The figure shows three views and two pictorial views of one solid part (mm, origin at its lowest corner). Answer the questions. Coordinates: 2 decimals unless noted, no trailing zeros. Write each loop counter-clockwise with the first axis right and the second up, starting at its lowest first coordinate (ties: lowest second). Pieces come first, ordered by that corner, then holes. Notation, with made-up numbers: (4, 7.25) - (33, 7.25) arc R29 cw to (33, 33.25) - close; hole circle Ø3 at (12, 72.25). An arc over 180 degrees is marked (long way). Use a Markdown table: item, result. Add a question column.
(1) Find the intervals of material crossed by line 1 (X direction, y = 6.25, z = 23) (1 decimal); line 2 (X direction, y = 1.5, z = 34.5); line 3 (Y direction, x = 40.5, z = 35.5), in increasing order. Write a range as from..to.
(2) For a pull along Z with two mould halves and no side action, classify the marked faces 1, 2, 3 and 4 as released by +Z, released by -Z, zero draft, split by the parting line, or undercut.
(3) The part is cut by section D-D, the plane z = 15. Give the vertices of the cut face in (x, y), then the cut area to 3 significant figures.
(4) Given pin 1 Ø3.5 at (x, z) = (17.02, 15.4) entering from -Y; pin 2 Ø1 at (x, z) = (36, 26) entering from +Y (3 decimals); pin 3 Ø3.5 at (x, z) = (29.15, 36.4) entering from +Y, each flat-ended and moving along its own axis, determine where each tip first touches the part or whether it passes through.
(5) The part is cut by section C-C, the plane x = 29.15. Give the vertices of the cut face in (y, z) (1 decimal), then the cut area to 3 significant figures.
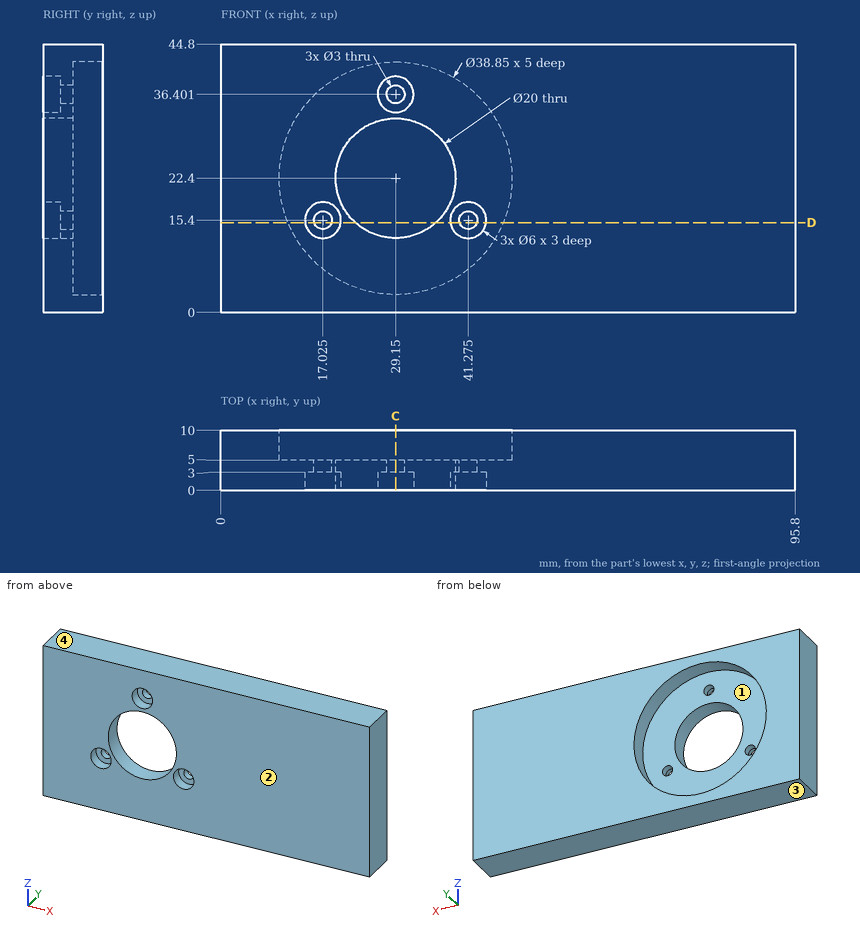
Model answer:
| question | item | result |
|---|---|---|
| 1 | line 1 | 0..9.7, 48.6..95.8 |
| 1 | line 2 | 0..26.83, 31.47..95.8 |
| 1 | line 3 | 0..5 |
| 2 | face 1 | undercut |
| 2 | face 2 | zero draft |
| 2 | face 3 | released by -Z |
| 2 | face 4 | released by +Z |
| 3 | outline | (0, 0) - (14.05, 0) - (14.05, 3) - (15.58, 3) - (15.58, 5) - (11.19, 5) - (11.19, 10) - (0, 10) - close; (18.47, 3) - (20, 3) - (20, 0) - (22.42, 0) - (22.42, 5) - (18.47, 5) - close; (35.88, 0) - (38.3, 0) - (38.3, 3) - (39.83, 3) - (39.83, 5) - (35.88, 5) - close; (42.72, 3) - (44.25, 3) - (44.25, 0) - (95.8, 0) - (95.8, 10) - (47.11, 10) - (47.11, 5) - (42.72, 5) - close |
| 3 | area | 664 mm^2 |
| 4 | pin 1 | y = 3 |
| 4 | pin 2 | through |
| 4 | pin 3 | y = 5 |
| 5 | outline | (0, 0) - (10, 0) - (10, 3) - (5, 3) - (5, 12.4) - (0, 12.4) - close; (0, 32.4) - (5, 32.4) - (5, 34.9) - (3, 34.9) - (3, 33.4) - (0, 33.4) - close; (0, 39.4) - (3, 39.4) - (3, 37.9) - (5, 37.9) - (5, 41.8) - (10, 41.8) - (10, 44.8) - (0, 44.8) - close |
| 5 | area | 130 mm^2 |
